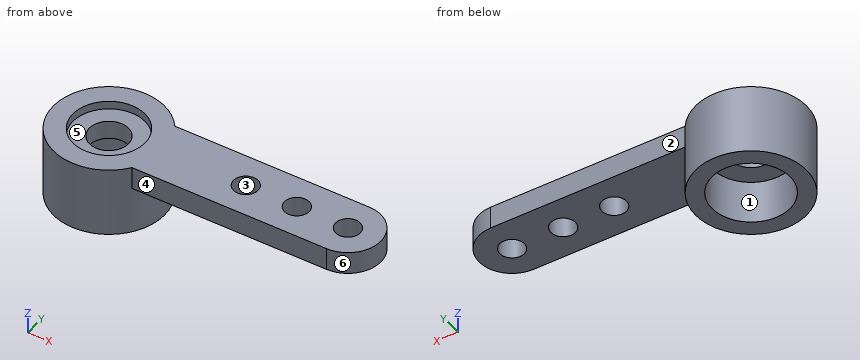
Autodesk Inventor part; units mm, degrees
ref_plane "YZ Plane" through (0, 0, 0) normal (1, 0, 0) x (0, 1, 0)
ref_plane "XZ Plane" through (0, 0, 0) normal (0, 1, 0) x (-1, 0, 0)
ref_plane "XY Plane" through (0, 0, 0) normal (0, 0, 1) x (1, 0, 0)
sketch "スケッチ1" plane through (0, 0, 0) normal (0, 0, 1) x (1, 0, 0)
  circle A0 centre (0, 0) radius 2.7
  circle A1 centre (0, 0) radius 0.95
  dimension "d0" = 5.4
  dimension "d1" = 1.9
extrude "押し出し1" add sketch "スケッチ1" along normal blind 3.4
sketch "スケッチ2" plane through (0, 0, 3.4) normal (0, 0, 1) x (1, 0, 0)
  circle A0 centre (0, 0) radius 1.75
  dimension "d4" = 3.5
extrude "押し出し2" cut sketch "スケッチ2" against normal blind 0.4
sketch "スケッチ3" plane through (0, 0, 0) normal (0, 0, -1) x (-1, 0, 0)
  circle A0 centre (0, 0) radius 0.95
  circle A1 centre (0, 0) radius 1.9
  dimension "d7" = 3.8
extrude "押し出し3" cut sketch "スケッチ3" against normal blind 2.1
sketch "スケッチ4" plane through (0, 0, 3.4) normal (0, 0, 1) x (1, 0, 0)
  arc A0 (11.7, -1.6) -> (11.7, 1.6) centre (11.7, 0) ccw
  line L0 (11.7, 1.6) -> (2.1749, 1.6)
  circle A1 centre (0, 0) radius 2.7
  line L1 (11.7, -1.6) -> (2.1749, -1.6)
  circle A2 centre (0, 0) radius 2.7
  arc A3 (2.1749, -1.6) -> (2.1749, 1.6) centre (0, 0) ccw
  dimension "d10" = 11.7
  dimension "d11" = 3.2
extrude "押し出し4" add sketch "スケッチ4" against normal blind 1.1 contours L1 A1 L0 A0
sketch "スケッチ5" plane through (0, 0, 3.4) normal (0, 0, 1) x (1, 0, 0)
  arc A0 (11.7, -1.6) -> (11.7, 1.6) centre (11.7, 0) ccw
  circle A1 centre (11.7, 0) radius 0.6
  circle A2 centre (9.2, 0) radius 0.6
  circle A3 centre (6.7, 0) radius 0.6
  point P0 (0, 0)
  dimension "d14" = 1.2
  dimension "d15" = 2.5
  dimension "d16" = 2.5
extrude "押し出し5" cut sketch "スケッチ5" against normal up to next
properties part number "hone"
Input: part model. Units: mm. Frame: model coordinates. Face numbers are marked on the shaded views. A direction names the side the tool comes from. Give positions to 0.01 mm unless a question says otherwise; leave off trailing zeros. Order: outer loops, then holes, each group sorted by start corner. A loop starts at its lowest first (then second) coordinate and runs counter-clockwise, first axis right, second up.
1. Pin query (flat end, axial travel): pin 1 Ø1 at (x, y) = (6, -1) entering from -Z; pin 2 Ø1 at (x, y) = (-0.5, -1) entering from +Z; pin 3 Ø1.2 at (x, z) = (9, 2.5) entering from -Y. Return the tip coordinate at first contact, or that it passes through.
Computed:
pin 1: stops at z = 2.3
pin 2: stops at z = 3
pin 3: stops at y = -1.6
2. Draft query along Y for the marked faces 4, 5 and 6. Return one class per face: released by +Y, released by -Y, zero draft, split by the parting line, or undercut.
Computed:
face 4: released by -Y
face 5: undercut
face 6: split by the parting line
3. Set-up query: the marked faces 1, 2 and 3. Return all of +Z, -Z, +X, -X, +Y, -Y with unobstructed straight access to the full face (end or side cutting, diameter ignored); none if empty.
Computed:
face 1: -Z
face 2: +Z, -Z, +X, +Y
face 3: +Z, -Z
4. Cut plane D-D (x = 9.2). Return loops of the section in (y, z).
Computed:
outline: (-1.6, 2.3) - (-0.6, 2.3) - (-0.6, 3.4) - (-1.6, 3.4) - close; (0.6, 2.3) - (1.6, 2.3) - (1.6, 3.4) - (0.6, 3.4) - close
5. Cut plane C-C (z = 2.55). Return loops of the section in (x, y).
Computed:
outline: (2.17, -1.6) - (11.7, -1.6) arc R1.6 ccw to (11.7, 1.6) - (2.17, 1.6) arc R2.7 ccw (long way) to start; hole circle Ø1.9 at (0, 0); hole circle Ø1.2 at (6.7, 0); hole circle Ø1.2 at (9.2, 0); hole circle Ø1.2 at (11.7, 0)
6. Cut plane B-B (x = 0). Return loops of the section in (y, z), and give its area (3 significant figures).
Computed:
outline: (-2.7, 0) - (-1.9, 0) - (-1.9, 2.1) - (-0.95, 2.1) - (-0.95, 3) - (-1.75, 3) - (-1.75, 3.4) - (-2.7, 3.4) - close; (0.95, 2.1) - (1.9, 2.1) - (1.9, 0) - (2.7, 0) - (2.7, 3.4) - (1.75, 3.4) - (1.75, 3) - (0.95, 3) - close
area: 7.27 mm2
7. Line query: probe 1 along Y at (x, z) = (9.2, 2.8); probe 2 along Y at (x, z) = (2.5, 2.85); probe 3 along Y at (x, z) = (0, 2.55). Output: solid intervals per line, ascending.
Computed:
probe 1: y = -1.6 to -0.6, 0.6 to 1.6
probe 2: y = -1.6 to 1.6
probe 3: y = -2.7 to -0.95, 0.95 to 2.7
8. Cut plane A-A (y = 0). State how many separate pieces and enclosed holes the cut face has, and give its area (3 significant figures).
Computed:
separate pieces: 5
enclosed holes: 0
area: 15.0 mm2
